The model under review builds one solid part; all positions refer to its coordinate system, in mm. Give positions to 0.01 mm unless a question says otherwise; leave off trailing zeros. Order: outer loops, then holes, each group sorted by start corner. A loop starts at its lowest first (then second) coordinate and runs counter-clockwise, first axis right, second up. Notation, with made-up numbers: (18.25, 41.25) - (31.25, 41.25) arc R7 ccw to (31.25, 51.25) - close; hole circle Ø11 at (17.5, 44). An arc over 180 degrees is marked (long way). Use CSV: the item, a comma, the result in double quotes.
```python
from build123d import *

# Parameters (mm, degrees)
ESQUISSE1_W              = 340
ESQUISSE1_H              = 260
BOSS_EXTRU_1_DEPTH       = 6
CONG_1_R                 = 60
ESQUISSE14_W             = 180
ESQUISSE14_H             = 10
ENL_V_MAT_EXTRU_7_DEPTH  = 10
ESQUISSE15_W             = 120
ESQUISSE15_H             = 2
ENL_V_MAT_EXTRU_8_DEPTH  = 10
CONG_2_R                 = 10
CONG_3_R                 = 8
ENL_V_MAT_EXTRU_10_DEPTH = 10
ESQUISSE18_W             = 8
ESQUISSE18_H             = 6
ENL_V_MAT_EXTRU_11_DEPTH = 10
ENL_V_MAT_EXTRU_13_DEPTH = 6
ENL_V_MAT_EXTRU_14_DEPTH = 10
ESQUISSE21_W             = 95
ESQUISSE21_H             = 171.650635095
ENL_V_MAT_EXTRU_15_DEPTH = 10
BOSS_EXTRU_3_DEPTH       = 6
ENL_V_MAT_EXTRU_18_DEPTH = 6
ESQUISSE25_W             = 8
ESQUISSE25_H             = 3
ENL_V_MAT_EXTRU_17_DEPTH = 6
ESQUISSE30_W             = 9
ESQUISSE30_H             = 171.650635095
BOSS_EXTRU_4_DEPTH       = 6
ESQUISSE32_W             = 6
ESQUISSE32_H             = 15
ESQUISSE32_H_2           = 15.174682453
ENL_V_MAT_EXTRU_19_DEPTH = 6
ESQUISSE33_R             = 2
ENL_V_MAT_EXTRU_20_DEPTH = 364.527165422


with BuildPart() as part:
    # Esquisse1 → Boss.-Extru.1 (new body)
    with BuildSketch(Plane.XY):
        with Locations((-170, 130)):
            Rectangle(ESQUISSE1_W, ESQUISSE1_H)
    extrude(amount=-BOSS_EXTRU_1_DEPTH)

    # Congé1
    cong_1_edges = [part.edges().sort_by_distance(p)[0] for p in [
        (0, 0, -3),
        (-340, 0, -3),
    ]]
    fillet(cong_1_edges, radius=CONG_1_R)

    # Esquisse14 → Enlèv. mat.-Extru.7 (cut)
    with BuildSketch(Plane(origin=(0, 0, -6), x_dir=(-1, 0, 0), z_dir=(0, 0, -1))):
        with Locations((235, 255)):
            Rectangle(ESQUISSE14_W, ESQUISSE14_H)
    extrude(amount=-ENL_V_MAT_EXTRU_7_DEPTH, mode=Mode.SUBTRACT)

    # Esquisse15 → Enlèv. mat.-Extru.8 (cut)
    with BuildSketch(Plane.XY):
        with Locations((-250, 249)):
            Rectangle(ESQUISSE15_W, ESQUISSE15_H)
    extrude(amount=-ENL_V_MAT_EXTRU_8_DEPTH, mode=Mode.SUBTRACT)

    # Congé2
    # the kernel refuses this fillet: 10 mm, written as the material it takes off along each edge
    with BuildSketch(Plane(origin=(-190, 250, 15), x_dir=(1, 0, 0), z_dir=(0, 0, -1))) as cong_2_piece_1:
        with BuildLine():
            CenterArc((6, 10), CONG_2_R, 233.130102354, 36.869897646)
            Line((0, 2), (-0.12, 1.84))
            ThreePointArc((-0.12, 1.84), (-0.2, 1), (-0.2, 0))
            Line((-0.2, 0), (0, -0.2))
            Line((0, -0.2), (6, -0.2))
            Line((6, -0.2), (6, 0))
        make_face()
    extrude(amount=36, mode=Mode.SUBTRACT)
    with BuildSketch(Plane(origin=(-310, 250, 15), x_dir=(0, -1, 0), z_dir=(0, 0, -1))) as cong_2_piece_2:
        with BuildLine():
            CenterArc((10, 6), CONG_2_R, 180, 36.869897646)
            Line((0, 6), (-0.2, 6))
            Line((-0.2, 6), (-0.2, 0))
            Line((-0.2, 0), (0, -0.2))
            ThreePointArc((0, -0.2), (1, -0.2), (1.84, -0.12))
            Line((1.84, -0.12), (2, 0))
        make_face()
    extrude(amount=36, mode=Mode.SUBTRACT)

    # Congé3
    cong_3_edges = [part.edges().sort_by_distance(p)[0] for p in [
        (-145, 260, -3),
        (-325, 260, -3),
    ]]
    fillet(cong_3_edges, radius=CONG_3_R)

    # Esquisse17 → Enlèv. mat.-Extru.10 (cut)
    with BuildSketch(Plane.XY):
        Polygon((-29.216285169, 245.39755551), (-23.478456633, 247.151785738), (-25.817430271, 254.802223786), (-31.555258806, 253.047993558), align=None)
        Polygon((-23.368851074, 226.271460391), (-17.631022538, 228.025690619), (-19.969996176, 235.676128667), (-25.707824712, 233.921898438), align=None)
        Polygon((-17.52141698, 207.145365271), (-11.783588444, 208.8995955), (-14.122562082, 216.550033547), (-19.860390617, 214.795803319), align=None)
        Polygon((-180, 150), (-30, 150), (-2.720065597, 179.254148065), (-9.568281369, 188.663047712), (-5.936154349, 189.77350038), (-8.275127987, 197.423938428), (-14.012956523, 195.6697082), (-13.538488979, 194.117794792), (-102.15398245, 315.868381088), (-205, 193.301270189), align=None)
    extrude(amount=-ENL_V_MAT_EXTRU_10_DEPTH, mode=Mode.SUBTRACT)

    # Esquisse18 → Enlèv. mat.-Extru.11 (cut)
    with BuildSketch(Plane.XY):
        with Locations((-110, 3)):
            Rectangle(ESQUISSE18_W, ESQUISSE18_H)
        with Locations((-130, 3)):
            Rectangle(ESQUISSE18_W, ESQUISSE18_H)
        with Locations((-150, 3)):
            Rectangle(ESQUISSE18_W, ESQUISSE18_H)
        with Locations((-170, 3)):
            Rectangle(ESQUISSE18_W, ESQUISSE18_H)
        with Locations((-190, 3)):
            Rectangle(ESQUISSE18_W, ESQUISSE18_H)
        with Locations((-210, 3)):
            Rectangle(ESQUISSE18_W, ESQUISSE18_H)
        with Locations((-230, 3)):
            Rectangle(ESQUISSE18_W, ESQUISSE18_H)
    extrude(amount=-ENL_V_MAT_EXTRU_11_DEPTH, mode=Mode.SUBTRACT)

    # Esquisse19 → Enlèv. mat.-Extru.13 (cut)
    with BuildSketch(Plane.XY):
        Polygon((-27.406549935, 260), (-61.490489073, 260), (-13.538488979, 194.117794792), (-14.012956523, 195.6697082), (-8.275127987, 197.423938428), (-5.936154349, 189.77350038), (-9.568281369, 188.663047712), (-2.720065597, 179.254148065), (0, 179.254148065), (0, 193.164126288), (0, 260), align=None)
        Polygon((-19.860390617, 214.795803319), (-14.122562082, 216.550033547), (-11.783588444, 208.8995955), (-17.52141698, 207.145365271), align=None, mode=Mode.SUBTRACT)
        Polygon((-25.707824712, 233.921898438), (-19.969996176, 235.676128667), (-17.631022538, 228.025690619), (-23.368851074, 226.271460391), align=None, mode=Mode.SUBTRACT)
        Polygon((-23.478456633, 247.151785738), (-29.216285169, 245.39755551), (-31.555258806, 253.047993558), (-25.817430271, 254.802223786), align=None, mode=Mode.SUBTRACT)
    extrude(amount=-ENL_V_MAT_EXTRU_13_DEPTH, mode=Mode.SUBTRACT)

    # Esquisse20 → Enlèv. mat.-Extru.14 (cut)
    with BuildSketch(Plane.XY):
        Polygon((-192.5, 171.650635095), (-340, 171.650635095), (-340, 260), (-157.424116728, 260.642727797), (-157.424116728, 250), align=None)
    extrude(amount=-ENL_V_MAT_EXTRU_14_DEPTH, mode=Mode.SUBTRACT)

    # Esquisse21 → Enlèv. mat.-Extru.15 (cut)
    with BuildSketch(Plane.XY):
        with Locations((-292.5, 85.825317548)):
            Rectangle(ESQUISSE21_W, ESQUISSE21_H)
    extrude(amount=-ENL_V_MAT_EXTRU_15_DEPTH, mode=Mode.SUBTRACT)

    # Esquisse27 → Boss.-Extru.3 (add)
    with BuildSketch(Plane.XY):
        Polygon((0, 179.254148065), (0, 194.58294763), (-20, 260), (-40, 260), (-192.5, 171.650635095), (-180, 150), (-30, 150), align=None)
    extrude(amount=-BOSS_EXTRU_3_DEPTH)

    # Esquisse29 → Enlèv. mat.-Extru.18 (cut)
    with BuildSketch(Plane.XY):
        Polygon((-40, 260), (-16.342847445, 182.620940619), (-26.572822846, 171.650635095), (-192.5, 171.650635095), align=None)
    extrude(amount=-ENL_V_MAT_EXTRU_18_DEPTH, mode=Mode.SUBTRACT)

    # Esquisse25 → Enlèv. mat.-Extru.17 (cut)
    with BuildSketch(Plane.XY):
        with Locations((-124, 151.5)):
            Rectangle(ESQUISSE25_W, ESQUISSE25_H)
        with Locations((-104, 151.5)):
            Rectangle(ESQUISSE25_W, ESQUISSE25_H)
        with Locations((-84, 151.5)):
            Rectangle(ESQUISSE25_W, ESQUISSE25_H)
        with Locations((-64, 151.5)):
            Rectangle(ESQUISSE25_W, ESQUISSE25_H)
        with Locations((-44, 151.5)):
            Rectangle(ESQUISSE25_W, ESQUISSE25_H)
        Polygon((-32.225134911, 152.012672503), (-28.133144751, 156.400794713), (-25.939083646, 154.354799632), (-30.031073806, 149.966677423), align=None)
        Polygon((-20.63116279, 164.44568543), (-18.437101685, 162.39969035), (-14.345111525, 166.78781256), (-16.53917263, 168.83380764), align=None)
        Polygon((-6.843129564, 174.832703278), (-9.037190669, 176.878698358), (-4.945200508, 181.266820568), (-2.751139404, 179.220825487), align=None)
        Polygon((-9.038404375, 194.655087151), (-6.169490107, 195.532202265), (-3.830516469, 187.881764218), (-6.699430737, 187.004649103), align=None)
        Polygon((-9.677950563, 207.007859337), (-12.546864831, 206.130744223), (-14.885838469, 213.78118227), (-12.016924201, 214.658297384), align=None)
        Polygon((-18.394298926, 225.256839342), (-15.525384658, 226.133954456), (-17.864358296, 233.784392504), (-20.733272563, 232.90727739), align=None)
        Polygon((-21.372818752, 245.260049575), (-23.71179239, 252.910487623), (-26.580706658, 252.033372509), (-24.24173302, 244.382934461), align=None)
    extrude(amount=-ENL_V_MAT_EXTRU_17_DEPTH, mode=Mode.SUBTRACT)

    # Esquisse30 → Boss.-Extru.4 (add)
    with BuildSketch(Plane.XY):
        with Locations((-249.5, 85.825317548)):
            Rectangle(ESQUISSE30_W, ESQUISSE30_H)
    extrude(amount=-BOSS_EXTRU_4_DEPTH)

    # Esquisse32 → Enlèv. mat.-Extru.19 (cut)
    with BuildSketch(Plane.XY):
        with Locations((-251, 128.5)):
            Rectangle(ESQUISSE32_W, ESQUISSE32_H)
        with Locations((-251, 93.412658773)):
            Rectangle(ESQUISSE32_W, ESQUISSE32_H_2)
        with Locations((-251, 58.5)):
            Rectangle(ESQUISSE32_W, ESQUISSE32_H)
        with Locations((-251, 23.5)):
            Rectangle(ESQUISSE32_W, ESQUISSE32_H)
    extrude(amount=-ENL_V_MAT_EXTRU_19_DEPTH, mode=Mode.SUBTRACT)

    # Esquisse33 → Enlèv. mat.-Extru.20 (cut, through all)
    with BuildSketch(Plane.XY):
        with Locations((-200, 3)):
            Circle(ESQUISSE33_R)
        with Locations((-140, 3)):
            Circle(ESQUISSE33_R)
        with Locations((-251, 41)):
            Circle(ESQUISSE33_R)
        with Locations((-251, 111)):
            Circle(ESQUISSE33_R)
    extrude(amount=-ENL_V_MAT_EXTRU_20_DEPTH, mode=Mode.SUBTRACT)


solid = part.part
```
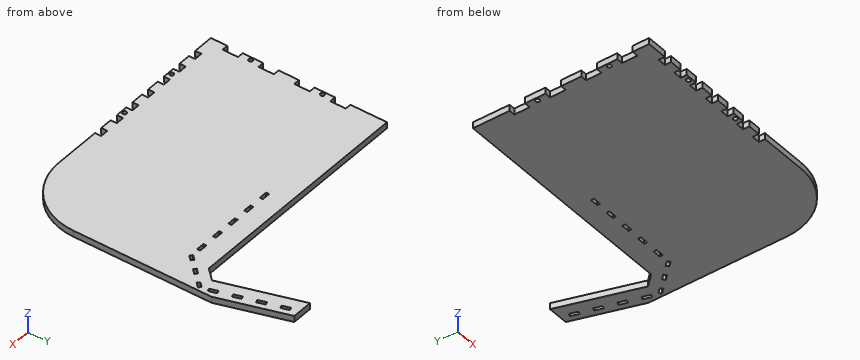
Item 1: Take a section at A-A, the plane z = -0.95. State how many separate pieces and enclosed holes the cut face has, and give its area (3 significant figures).
Results list:
separate pieces,"1"
enclosed holes,"16"
area,"43,600 mm2"
Item 2: Wall thickness on L1, parallel to Y at x = -66, z = -0.65; L2, parallel to Y at x = -200, z = -2.8; L3, parallel to X at y = 130, z = -1.55: over which ranges is each line inside the solid? List them lowest first.
Results list:
L1,"y = 0 to 150, 153 to 171.65"
L2,"y = 0 to 1, 5 to 171.65"
L3,"x = -248 to 0"
Item 3: Clearance check with flat-ended pins moving along their axes: pin 1 (3 mm diameter, centred on y = 28, z = -1.5, fed in from -X); pin 2 (1.8 mm diameter, centred on x = -108.5, z = -3, fed in from -Y); pin 3 (3 mm diameter, centred on x = -122, z = -4.5, fed in from +Y). State where each tip first meets the part, or that it passes through.
Results list:
pin 1,"stops at x = -248"
pin 2,"stops at y = 6"
pin 3,"stops at y = 171.65"
Item 4: Take a section at C-C, the plane y = 35. Give the boundary of the cut face in (x, z), and give its area (3 significant figures).
Results list:
outline,"(-254, -6) - (-5.46, -6) - (-5.46, 0) - (-254, 0) - close"
area,"1,490 mm2"
Item 5: Take a section at B-B, the plane x = -74. Give the boundary of the cut face in (y, z).
Results list:
outline,"(0, -6) - (171.65, -6) - (171.65, 0) - (0, 0) - close"
